Build history of the part. All positions in model axes, mm. A direction names the side the tool comes from. Coordinates: 2 decimals unless noted, no trailing zeros. Loops run counter-clockwise (first coordinate to the right, second up) from the corner with the lowest first, then second, coordinate; pieces in that order, holes last. Notation, with made-up numbers: M -12.5,73.25 L 24.5,73.25 A16 cw 24.5,94.25 Z; hole C 6,-16 d10. An arc over 180 degrees is marked long. Write each question's results on one line, items separated by ' | '. Start each with the question number.
from build123d import *
from OCP.BRepFilletAPI import BRepFilletAPI_MakeChamfer

# Parameters (mm, degrees)
SKETCH_1_W          = 30
SKETCH_1_H          = 150
SKETCH_1_R          = 1.6
EXTRUDE_1_DEPTH     = 3
CUT_EXTRUDE_3_REACH = 149.17
SKETCH_4_W          = 5
SKETCH_4_H          = 55
CHAMFER_1_SIZE      = 2.5
CUT_EXTRUDE_4_REACH = 149.17
SKETCH_5_R          = 2.55
EXTRUDE_5_DEPTH     = 3
EXTRUDE_2_DEPTH     = 3
FILLET_2_R          = 65
FILLET_3_R          = 115
FILLET_4_R          = 5
CUT_EXTRUDE_START   = -3
CUT_EXTRUDE_6_DEPTH = 3
CHAMFER_2_SIZE      = 3
CHAMFER_2_SIZE2     = 2.901779002


# Read off the part's stored shape, not the designer's step: 切除-拉伸6
with BuildPart() as part:
    # 草图1 → 凸台-拉伸1 (new body)
    with BuildSketch(Plane.XY):
        with Locations((10, -70)):
            Rectangle(SKETCH_1_W, SKETCH_1_H)
        Circle(SKETCH_1_R, mode=Mode.SUBTRACT)
        with Locations((20, 0)):
            Circle(SKETCH_1_R, mode=Mode.SUBTRACT)
    extrude(amount=EXTRUDE_1_DEPTH)

    # 草图4 → 切除-拉伸3 (cut, up to next)
    with BuildSketch(Plane.XY.offset(3), mode=Mode.PRIVATE) as cut_extrude_3_sk1:
        with Locations((-2.5, -117.5)):
            Rectangle(SKETCH_4_W, SKETCH_4_H)
    cut_extrude_3_tool1 = extrude(cut_extrude_3_sk1.sketch, amount=-CUT_EXTRUDE_3_REACH, mode=Mode.PRIVATE) & part.part
    add(cut_extrude_3_tool1.solids().sort_by_distance((-2.5, -117.5, 3))[0], mode=Mode.SUBTRACT)

    # 倒角1
    chamfer_1_edges = [part.edges().sort_by_distance(p)[0] for p in [
        (-5, -90, 1.5),
    ]]
    chamfer(chamfer_1_edges, length=CHAMFER_1_SIZE)

    # 草图5 → 切除-拉伸4 (cut, up to next)
    with BuildSketch(Plane.XY.offset(3), mode=Mode.PRIVATE) as cut_extrude_4_sk1:
        with Locations((12.5, -140)):
            Circle(SKETCH_5_R)
    cut_extrude_4_tool1 = extrude(cut_extrude_4_sk1.sketch, amount=-CUT_EXTRUDE_4_REACH, mode=Mode.PRIVATE) & part.part
    add(cut_extrude_4_tool1.solids().sort_by_distance((12.5, -140, 3))[0], mode=Mode.SUBTRACT)

    # 草图9 → 凸台-拉伸5 (add)
    with BuildSketch(Plane(origin=(0, 0, 0), x_dir=(-1, 0, 0), z_dir=(0, 0, -1))):
        Polygon((5, -87.5), (0, -117.5), (0, -90), (2.5, -90), align=None)
    extrude(amount=-EXTRUDE_5_DEPTH)

    # 草图11 → 拉伸-薄壁2 (add)
    with BuildSketch(Plane.XY.offset(3)):
        Polygon((19.5, -67.916286439), (19.5, -61.710608008), (19.5, -3.420169007), (16.5, -3.420169007), (16.5, -61.710608008), (16.5, -67.916286439), align=None)
    extrude(amount=-EXTRUDE_2_DEPTH)

    # 圆角2
    fillet_2_edges = [part.edges().sort_by_distance(p)[0] for p in [
        (-5, -87.5, 1.5),
    ]]
    fillet(fillet_2_edges, radius=FILLET_2_R)

    # 圆角3
    fillet_3_edges = [part.edges().sort_by_distance(p)[0] for p in [
        (0, -117.5, 1.5),
    ]]
    fillet(fillet_3_edges, radius=FILLET_3_R)

    # 圆角4
    fillet_4_edges = [part.edges().sort_by_distance(p)[0] for p in [
        (0, -145, 1.5),
    ]]
    fillet(fillet_4_edges, radius=FILLET_4_R)

    # 切除-拉伸6 outline → 切除-拉伸6 (cut)
    with BuildSketch(Plane.XY.offset(3).offset(CUT_EXTRUDE_START)):
        with BuildLine():
            ThreePointArc((19.997033519, -140.172209208), (18.47411528, -143.595903644), (15, -145))
            Line((15, -145), (25, -145))
            Line((25, -145), (25, 5))
            Line((25, 5), (19.997033519, -140.172209208))
        make_face()
        with BuildLine():
            ThreePointArc((10, -145), (6.464466094, -143.535533906), (5, -140))
            Line((5, -140), (5, -83.1053734))
            ThreePointArc((5, -83.1053734), (2.483450387, -52.175255091), (-5, -22.058761091))
            Line((-5, -22.058761091), (-5, -82.120435531))
            ThreePointArc((-5, -82.120435531), (-4.778523942, -87.481670081), (-4.115605049, -92.806369705))
            Line((-4.115605049, -92.806369705), (-1.564698759, -108.111807444))
            ThreePointArc((-1.564698759, -108.111807444), (-0.391842257, -117.532429856), (0, -127.017690984))
            Line((0, -127.017690984), (0, -140))
            ThreePointArc((0, -140), (1.464466094, -143.535533906), (5, -145))
            Line((5, -145), (10, -145))
        make_face()
    extrude(amount=CUT_EXTRUDE_6_DEPTH, mode=Mode.SUBTRACT)

    # 倒角2: one chamfer whose edges measure the first distance from different faces: ONE call of the kernel's chamfer builder (chamfer() names one face for all edges)
    chamfer_2_edges_1 = [part.edges().sort_by_distance(p)[0] for p in [
        (-5, 5, 1.5),
    ]]
    chamfer_2_edges_2 = [part.edges().sort_by_distance(p)[0] for p in [
        (25, 5, 1.5),
    ]]
    chamfer_2_side_2 = [part.faces().sort_by_distance(p)[0] for p in [
        (22.498516759, -67.586104604, 1.5),
    ]]
    chamfer_2 = BRepFilletAPI_MakeChamfer(part.part.solid().wrapped)
    for e in chamfer_2_edges_1:
        chamfer_2.Add(CHAMFER_2_SIZE, e.wrapped)
    for e in chamfer_2_edges_2:
        chamfer_2.Add(CHAMFER_2_SIZE, CHAMFER_2_SIZE2, e.wrapped, chamfer_2_side_2[0].wrapped)  # the first distance lies on this face
    add(Compound.cast(chamfer_2.Shape()), mode=Mode.REPLACE)


solid = part.part
1. Which spindle directions (+Z, -Z, +X, -X, +Y, -Y) get a long thin tool onto all of the face, cutting with end or side? Do faces 1 (the flat face through (-3, 4, 1)), 2 (the flat face through (5, -112, 1)). Say none if no direction does.
2. Mould opens along Y. For faces 3 (the cylindrical face through (12.17, -137.47, 1.52)), 4 (the cylindrical face through (18.82, 1.08, 1.48)), 5 (the flat face through (23.5, 3.5, 1.5)), 6 (the cylindrical face through (2.553, -52.605, 1.479)) say: +Y half, -Y half, draft (parallel to the pull), parting line (faces both ways), or undercut.
3. Band-saw the part on B-B, the plane y = 0. List the corners of the cut face in (x, z), plus the area to 3 significant figures.
4. Band-saw the part on D-D, the plane y = -45. List the corners of the cut face in (x, z).
5. Pin check, flat tips, straight feed: pin 1 (4.5 mm diameter, centred on x = 12.5, y = -140, fed in from -Z); pin 2 (1 mm diameter, centred on y = -51.5, z = 2.5, fed in from -X); pin 3 (0.9 mm diameter, centred on y = -100, z = 1.5, fed in from -X). Stop position of each tip, or through.
6. Wall check: line 1 along Y through (x, z) = (12.5, 2.25); line 2 along X through (y, z) = (-140, 1.3); line 3 along Y through (x, z) = (10.5, 0.5). Give the ranges that are in metal, low to high.
7. Band-saw the part on C-C, the plane x = 0. List the corners of the cut face in (y, z).
8. Band-saw the part on A-A, the plane x = 12.5. List the corners of the cut face in (y, z), plus the area to 3 significant figures.
Checked values:
1) face 1: +Z, -Z, -X, +Y | face 2: +Z, -Z, -X, -Y
2) face 3: undercut | face 4: undercut | face 5: +Y half | face 6: -Y half
3) outline: M -5,0 L -1.6,0 L -1.6,3 L -5,3 Z; M 1.6,0 L 18.4,0 L 18.4,3 L 1.6,3 Z; M 21.6,0 L 24.83,0 L 24.83,3 L 21.6,3 Z | area: 70.3 mm²
4) outline: M 1.17,0 L 23.28,0 L 23.28,3 L 1.17,3 Z
5) pin 1: through | pin 2: x = 2.29 | pin 3: x = 5
6) line 1: -145 to -142.55, -137.45 to 5 | line 2: 5 to 9.95, 15.05 to 20 | line 3: -145 to -141.58, -138.42 to 5
7) outline: M -39.65,0 L -1.6,0 L -1.6,3 L -39.65,3 Z; M 1.6,0 L 5,0 L 5,3 L 1.6,3 Z
8) outline: M -145,0 L -142.55,0 L -142.55,3 L -145,3 Z; M -137.45,0 L 5,0 L 5,3 L -137.45,3 Z | area: 435 mm²
